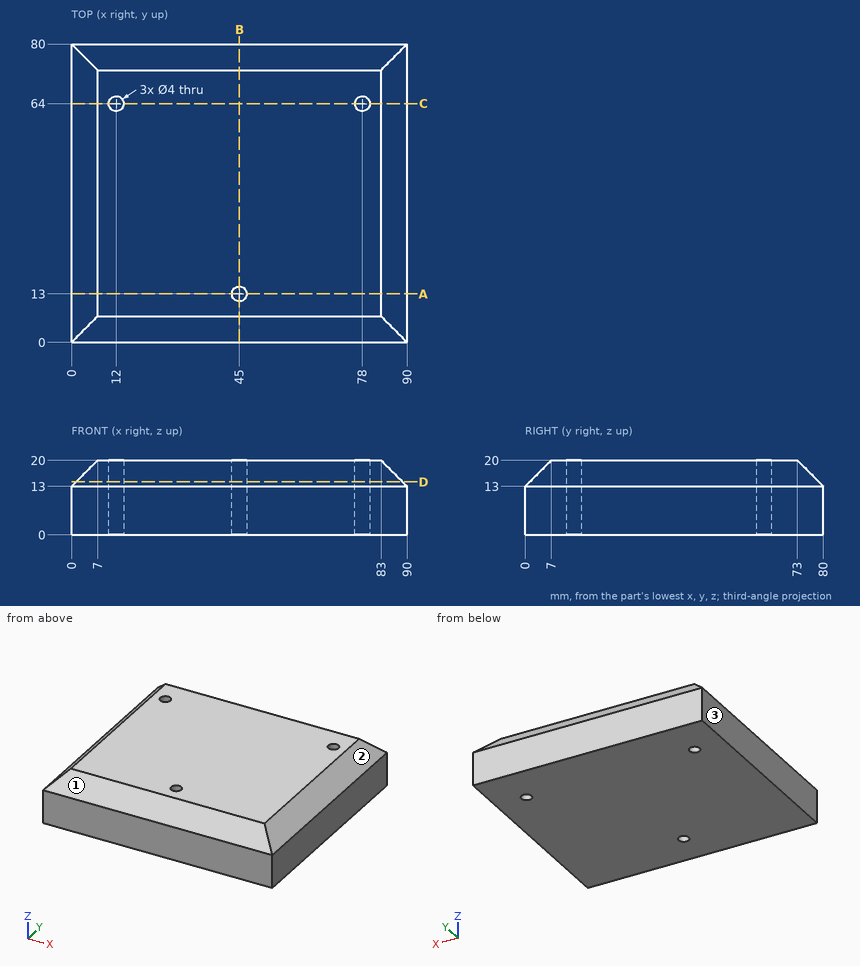
Answer from the drawing. Dimensions are ordinates in mm from the lowest x, y and z of the part. Coordinates: 2 decimals unless noted, no trailing zeros. Write each loop counter-clockwise with the first axis right and the second up, starting at its lowest first coordinate (ties: lowest second). Pieces come first, ordered by that corner, then holes. Notation, with made-up numbers: M -28.75,71.5 L -19.75,71.5 A15 cw -19.75,99.5 Z; hole C 20,19.25 d6. An arc over 180 degrees is marked long. Use a Markdown table: item, result.
Q1. Straight lines are drawn through the part: L1, parallel to Y at x = 78, z = 10.5; L2, parallel to X at y = 64, z = 13.25; L3, parallel to Y at x = 45, z = 6. For each, find the intervals that lie inside material, in ascending order. Write a range as [from, to].
Answer block:
| item | result |
|---|---|
| L1 | y = [0, 62], [66, 80] |
| L2 | x = [0.25, 10], [14, 76], [80, 89.75] |
| L3 | y = [0, 11], [15, 80] |
Q2. The part is cut by section D-D, the plane z = 14.25. Write down the section's boundary in (x, y).
Answer block:
| item | result |
|---|---|
| outline | M 1.25,1.25 L 88.75,1.25 L 88.75,78.75 L 1.25,78.75 Z; hole C 12,64 d4; hole C 45,13 d4; hole C 78,64 d4 |
Q3. Each of these flat-tipped pins is pushed along its axis until it touches: pin 1 Ø10 at (x, y) = (19, 47.5) entering from -Z; pin 2 Ø3.5 at (x, y) = (12, 64) entering from -Z. Where does it stop, or does it pass through?
Answer block:
| item | result |
|---|---|
| pin 1 | stops at z = 0 |
| pin 2 | passes through |
Q4. Determine the mould class of the marked faces 1, 2 and 3 for opening direction X: released by +X, released by -X, zero draft, split by the parting line, or undercut.
Answer block:
| item | result |
|---|---|
| face 1 | zero draft |
| face 2 | released by +X |
| face 3 | released by -X |
Q5. The part is cut by section C-C, the plane y = 64. Write down the section's boundary in (x, z), then the cut area to 3 significant figures.
Answer block:
| item | result |
|---|---|
| outline | M 0,0 L 10,0 L 10,20 L 7,20 L 0,13 Z; M 14,0 L 76,0 L 76,20 L 14,20 Z; M 80,0 L 90,0 L 90,13 L 83,20 L 80,20 Z |
| area | 1,590 mm2 |
Q6. The part is cut by section A-A, the plane y = 13. Write down the section's boundary in (x, z).
Answer block:
| item | result |
|---|---|
| outline | M 0,0 L 43,0 L 43,20 L 7,20 L 0,13 Z; M 47,0 L 90,0 L 90,13 L 83,20 L 47,20 Z |
Q7. The part is cut by section B-B, the plane x = 45. Write down the section's boundary in (y, z).
Answer block:
| item | result |
|---|---|
| outline | M 0,0 L 11,0 L 11,20 L 7,20 L 0,13 Z; M 15,0 L 80,0 L 80,13 L 73,20 L 15,20 Z |
